Geometry check sheet. Reference: drawing and pictorial views, mm from the part's lowest x, y, z. Coordinates: 2 decimals unless noted, no trailing zeros. Write each loop counter-clockwise with the first axis right and the second up, starting at its lowest first coordinate (ties: lowest second). Pieces come first, ordered by that corner, then holes. Notation, with made-up numbers: M 41,78.25 L 58,78.25 A23 cw 58,105.25 Z; hole C 64.5,35 d6. An arc over 180 degrees is marked long. One line per item, written item: value.
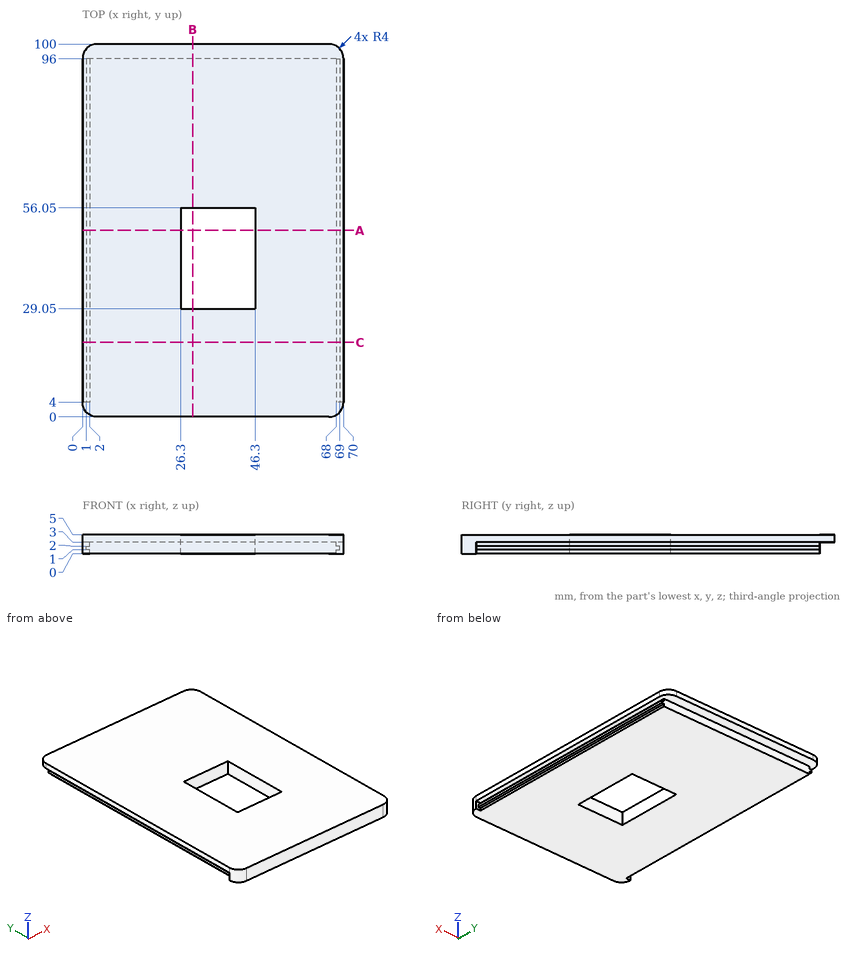
Item 1: Go/stop test with flat-tipped pins: P1, Ø1.5, axis at y = 38, z = 1.5, coming from the -X side; P2, Ø0.8, axis at x = 68.5, y = 51.5, coming from the -Z side; P3, Ø0.5, axis at y = 52, z = 2.5, coming from the -X side. Record where each tip stops, or that it passes through.
The answers:
P1: stops at x = 1
P2: stops at z = 1
P3: stops at x = 2
Item 2: Cross-section at B-B, the plane x = 29.5. Enter the section's corners in (y, z), and give its area (3 significant figures).
The answers:
outline: M 0,0 L 29.05,0 L 29.05,5 L 0,5 Z; M 56.05,0 L 96,0 L 96,3 L 100,3 L 100,5 L 56.05,5 Z
area: 353 mm²
Item 3: Cross-section at A-A, the plane y = 50. Enter the section's corners in (x, z).
The answers:
outline: M 0,3 L 2,3 L 2,2 L 1,2 L 1,1 L 2,1 L 2,0 L 26.3,0 L 26.3,5 L 0,5 Z; M 46.3,0 L 68,0 L 68,1 L 69,1 L 69,2 L 68,2 L 68,3 L 70,3 L 70,5 L 46.3,5 Z
Item 4: Scan lines: line 1 (Y direction, x = 46, z = 1.05); line 2 (Y direction, x = 61, z = 0.55); line 3 (Y direction, x = 46, z = 4.55). Record each from-to range of solid material in increasing order.
The answers:
line 1: y = 0 to 29.05, 56.05 to 96
line 2: y = 0 to 96
line 3: y = 0 to 29.05, 56.05 to 100
Item 5: Cross-section at C-C, the plane y = 20. Enter the section's corners in (x, z).
The answers:
outline: M 0,3 L 2,3 L 2,2 L 1,2 L 1,1 L 2,1 L 2,0 L 68,0 L 68,1 L 69,1 L 69,2 L 68,2 L 68,3 L 70,3 L 70,5 L 0,5 Z
